from build123d import *

# Parameters (mm, degrees)
F0_W        = 149.9416083097
F0_H        = 15.8279500902
F1_DEPTH    = 4.826
F2_SIZE     = 5
F3_T1_DEPTH = 164.9264657238
F4_T1_DEPTH = 164.9264657238
F5_T1_DEPTH = 30.8128075042


# Not quite as in the source:
# - a fillet or chamfer that OpenCascade refuses, or shapes differently, is made with other operations: its cross-section is extruded or revolved along the edge and cut away or added


with BuildPart() as f1:
    # F0 (on Top) → F1 (new body)
    with BuildSketch(Plane.XY):
        with Locations((-74.9708041549, 7.9139750451)):
            Rectangle(F0_W, F0_H)
    extrude(amount=F1_DEPTH)

    # F2
    f2_edges = [f1.edges().sort_by_distance(p)[0] for p in [
        (-149.941608, 15.82795, 2.413),
        (-149.941608, 0, 2.413),
        (0, 15.82795, 2.413),
        (0, 0, 2.413),
    ]]
    chamfer(f2_edges, length=F2_SIZE)

    # F3: fillet of radius 5 on 1 edges, made by hand

    # F3_s2 → F3_t1 (cut)
    with BuildSketch(Plane.YZ.offset(-157.4340370168)):
        with BuildLine():
            ThreePointArc((0, 4.826), (1.5235005962, 1.4034738983), (4.9969714828, 0))
            Line((4.9969714828, 0), (0, 0))
            Line((0, 0), (0, 4.826))
        make_face()
    extrude(amount=F3_T1_DEPTH, mode=Mode.SUBTRACT)

    # F4: fillet of radius 5 on 1 edges, made by hand

    # F4_s2 → F4_t1 (cut)
    with BuildSketch(Plane.YZ.offset(-157.4340370168)):
        with BuildLine():
            ThreePointArc((15.8279500902, 4.826), (14.304449494, 1.4034738983), (10.8309786074, 0))
            Line((10.8309786074, 0), (15.8279500902, 0))
            Line((15.8279500902, 0), (15.8279500902, 4.826))
        make_face()
    extrude(amount=F4_T1_DEPTH, mode=Mode.SUBTRACT)

    # F5: fillet of radius 5 on 1 edges, made by hand

    # F5_s2 → F5_t1 (cut)
    with BuildSketch(Plane.XZ.offset(-23.3203787972)):
        with BuildLine():
            ThreePointArc((0, 4.826), (-1.5235005962, 1.4034738983), (-4.9969714828, 0))
            Line((-4.9969714828, 0), (0, 0))
            Line((0, 0), (0, 4.826))
        make_face()
    extrude(amount=F5_T1_DEPTH, mode=Mode.SUBTRACT)


solid = f1.part
The listing builds one solid part. Answer for the finished solid, in the listing's coordinates (mm). Coordinates: 2 decimals unless noted, no trailing zeros. Order: outer loops, then holes, each group sorted by start corner. A loop starts at its lowest first (then second) coordinate and runs counter-clockwise, first axis right, second up.
Q1. A cutting plane is placed at B-B, the plane x = -31.5. Write down the section's boundary in (y, z), and give its area (3 significant figures).
Q2. Consider line 1 (Z direction, x = -70, y = 11.5); line 2 (Y direction, x = -105, z = 1.6); line 3 (Y direction, x = -60, z = 0.55). Determine where each line is inside the solid, lowest interval first.
Q3. Given P1, Ø2, axis at x = -88.5, z = 1, coming from the +Y side; P2, Ø2, axis at y = 3.5, z = 4, coming from the -X side, each flat-ended and moving along its own axis, determine where each tip first touches the part or whether it passes through.
Q4. A cutting plane is placed at A-A, the plane z = 1.75. Write down the section's boundary in (x, y).
Answers follow:
1. outline: (0, 4.83) arc R5 ccw to (5, 0) - (10.83, 0) arc R5 ccw to (15.83, 4.83) - close
1. area: 65.7 mm2
2. line 1: z = 0.04 to 4.83
2. line 2: y = 1.33 to 14.5
2. line 3: y = 2.72 to 13.11
3. P1: stops at y = 14.83
3. P2: stops at x = -149.44
4. outline: (-149.94, 5) - (-146.14, 1.2) - (-3.8, 1.2) - (-1.2, 3.8) - (-1.2, 12.03) - (-3.8, 14.63) - (-146.14, 14.63) - (-149.94, 10.83) - close
